Input: dimensioned drawing with shaded views. Units: mm. Origin: part minimum x, y, z. A direction names the side the tool comes from. Coordinates: 2 decimals unless noted, no trailing zeros. Order: outer loops, then holes, each group sorted by start corner. A loop starts at its lowest first (then second) coordinate and runs counter-clockwise, first axis right, second up. Notation, with made-up numbers: (35, -16) - (47, -16) arc R14 ccw to (47, 3) - close; hole circle Ø2 at (-37.75, 1). An arc over 180 degrees is marked (long way). One line per question, with ' | ' between items. Start each with the question number.
(1) Section A-A (y = 14). Return the cut outline in (x, z), then the cut area to 3 significant figures.
(2) Contact query for a flat-ended pin moving along its axis: P1, Ø4.5, axis at x = 26.5, y = 9, coming from the -Z side. Output: stop coordinate, or through.
(3) Access query for the marked faces 4, 5 and 6. Directions: +Z, -Z, +X, -X, +Y, -Y. A direction counts if a zero-diameter tool reaches every point of the face in a straight line with its end or side. Return the directions, or none.
(4) Section C-C (y = 19.05). Return the cut outline in (x, z).
(5) Draft query along X for the marked faces 1, 2 and 3. Return one class per face: +X half, -X half, draft (parallel to the pull), parting line (faces both ways), or undercut.
(6) Line query: line 1 along X through (y, z) = (21, 20); line 2 along X through (y, z) = (28.5, 12.5); line 3 along Z through (x, y) = (28.5, 28). Output: solid intervals per line, ascending.
(7) Section B-B (z = 7.5). Return the cut outline in (x, y), then the cut area to 3 significant figures.
(8) Section D-D (x = 24). Return the cut outline in (y, z).
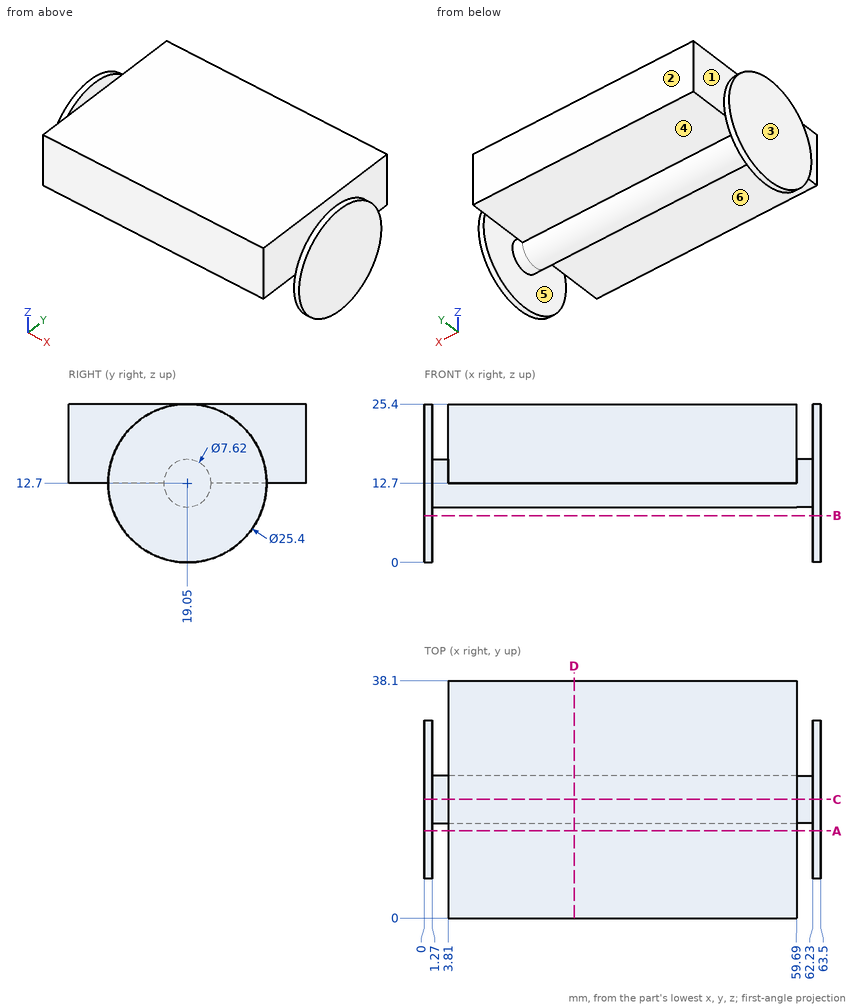
Response values:
1) outline: (0, 1.05) - (1.27, 1.05) - (1.27, 24.35) - (0, 24.35) - close; (3.81, 12.7) - (59.69, 12.7) - (59.69, 25.4) - (3.81, 25.4) - close; (62.23, 1.05) - (63.5, 1.05) - (63.5, 24.35) - (62.23, 24.35) - close | area: 769 mm²
2) P1: stops at z = 12.7
3) face 4: -Z, +Y | face 5: none | face 6: -Z, -Y
4) outline: (0, 0) - (1.27, 0) - (1.27, 8.89) - (62.23, 8.89) - (62.23, 0) - (63.5, 0) - (63.5, 25.4) - (62.23, 25.4) - (62.23, 16.51) - (59.69, 16.51) - (59.69, 25.4) - (3.81, 25.4) - (3.81, 16.51) - (1.27, 16.51) - (1.27, 25.4) - (0, 25.4) - close
5) face 1: undercut | face 2: draft | face 3: -X half
6) line 1: x = 0 to 1.27, 3.81 to 59.69, 62.23 to 63.5 | line 2: x = 0 to 1.27, 62.23 to 63.5 | line 3: z = 12.7 to 25.4
7) outline: (0, 7.46) - (1.27, 7.46) - (1.27, 30.64) - (0, 30.64) - close; (62.23, 7.46) - (63.5, 7.46) - (63.5, 30.64) - (62.23, 30.64) - close | area: 58.9 mm²
8) outline: (0, 12.7) - (15.24, 12.7) arc R3.81 ccw to (22.86, 12.7) - (38.1, 12.7) - (38.1, 25.4) - (0, 25.4) - close
